```python
from build123d import *

# Parameters (mm, degrees)
SKETCH1_R           = 2.25
BOSS_EXTRUDE1_DEPTH = 3.175


with BuildPart() as part:
    # Sketch1 → Boss-Extrude1 (new body)
    with BuildSketch(Plane.XY):
        Polygon((-214.3125, -34.925), (-214.3125, -88.9), (214.3125, -88.9), (214.3125, -34.925), (176.2125, -34.925), (176.2125, 22.225), (214.3125, 22.225), (214.3125, 88.9), (-214.3125, 88.9), (-214.3125, 22.225), (-176.2125, 22.225), (-176.2125, -34.925), align=None)
        with Locations((-192.0875, -63.5)):
            Circle(SKETCH1_R, mode=Mode.SUBTRACT)
        with Locations((192.0875, -63.5)):
            Circle(SKETCH1_R, mode=Mode.SUBTRACT)
        with Locations((-192.0875, 46.0375)):
            Circle(SKETCH1_R, mode=Mode.SUBTRACT)
        with Locations((192.0875, 46.0375)):
            Circle(SKETCH1_R, mode=Mode.SUBTRACT)
    extrude(amount=-BOSS_EXTRUDE1_DEPTH)


solid = part.part
```
Could you check a few things on this model? Use its own coordinates, in mm. Round coordinates to 2 decimals unless told otherwise and drop trailing zeros. Loops run counter-clockwise (first coordinate to the right, second up) from the corner with the lowest first, then second, coordinate; pieces in that order, holes last. Notation, with made-up numbers: (8.25, -1) - (13.25, -1) arc R23 ccw to (13.25, 12) - close; hole circle Ø7 at (25.5, 15.5). An arc over 180 degrees is marked (long way). Answer in a Markdown table with one row per item. Add a question column.
(1) I need wall thicknesses on line 1 along X through (y, z) = (13, -1.6); line 2 along Y through (x, z) = (188.5, -0.8) (3 decimals); line 3 along X through (y, z) = (44.5, -1). Which ranges of each line are inside material? Lowest first, please.
(2) If we section it at B-B (z = -1.3): State how many separate pieces and enclosed holes the cut face has, plus the area to 3 significant figures.
(3) If we section it at A-A (x = -182): Please give me the cut outline in (y, z) (3 decimals).
(4) I'm going to push a flat-ended pin straight in: pin 1 (1.6 mm diameter, centred on y = -17.5, z = -1.5, fed in from +X). Where does the tip first touch, or does it pass through?
(5) If we section it at C-C (y = -2.5): Please give me the cut outline in (x, z) (1 decimal).
Model answer:
| question | item | result |
|---|---|---|
| 1 | line 1 | x = -176.21 to 176.21 |
| 1 | line 2 | y = -88.9 to -34.925, 22.225 to 88.9 |
| 1 | line 3 | x = -214.31 to -193.73, -190.44 to 190.44, 193.73 to 214.31 |
| 2 | separate pieces | 1 |
| 2 | enclosed holes | 4 |
| 2 | area | 71,800 mm² |
| 3 | outline | (-88.9, -3.175) - (-34.925, -3.175) - (-34.925, 0) - (-88.9, 0) - close; (22.225, -3.175) - (88.9, -3.175) - (88.9, 0) - (22.225, 0) - close |
| 4 | pin 1 | stops at x = 176.21 |
| 5 | outline | (-176.2, -3.2) - (176.2, -3.2) - (176.2, 0) - (-176.2, 0) - close |
